Part model, mm, in its own coordinate system. Coordinates: 2 decimals unless noted, no trailing zeros. Order: outer loops, then holes, each group sorted by start corner. A loop starts at its lowest first (then second) coordinate and runs counter-clockwise, first axis right, second up.
1) Cut at C-C (z = 2). List the corners of the cut face in (x, y).
2) Cut at A-A (x = 0). List the corners of the cut face in (y, z), and give its area (3 significant figures).
3) Cut at D-D (y = -37.5). List the corners of the cut face in (x, z).
4) Pin check, flat tips, straight feed: pin 1 Ø3 at (x, z) = (-47.5, 5) entering from -Y (3 decimals); pin 2 Ø15 at (x, y) = (-76.2, 0) entering from +Z; pin 3 Ø3 at (x, z) = (31.5, 1) entering from -Y. Stop position of each tip, or through.
5) Cut at B-B (y = -4.5). List the corners of the cut face in (x, z).
6) Wall check: L1, parallel to Y at x = 0, z = 2.25; L2, parallel to X at y = 8.5, z = 5; L3, parallel to Y at x = -76.2, z = 4. Give the ranges that are in metal, low to high.
7) Mould opens along Y. For faces 1 (the cylindrical face through (-59.56, -34.48, 3.13)), 2 (the cylindrical face through (-59.14, 34.65, 3.13)), 3 (the flat face through (26, -41, 6.35)), 4 (the cylindrical face through (-64.086, 3.815, 3.131)) say: +Y half, -Y half, draft (parallel to the pull), parting line (faces both ways), or undercut.
```python
from build123d import *

# Parameters (mm, degrees)
F0_R     = 12.7
F0_R_2   = 44.45
F1_DEPTH = 6.35


# Not quite as in the source:
# - a length typed as a fraction of an inch, garbled in the dataset ("3 / 203.2 mm" for 3/8 in), is restored


with BuildPart() as f1:
    # F0 (on Top) → F1 (new body)
    with BuildSketch(Plane.XY):
        with BuildLine():
            ThreePointArc((-46.13671875, 43.6308741946), (-59.3475236203, 34.5646316236), (-75.1176136364, 31.7315448688))
            ThreePointArc((-75.1176136364, 31.7315448688), (-107.95, 0), (-75.1176136364, -31.7315448688))
            ThreePointArc((-75.1176136364, -31.7315448688), (-59.3475236203, -34.5646316236), (-46.13671875, -43.6308741946))
            ThreePointArc((-46.13671875, -43.6308741946), (-0.5192783502, -63.4978767361), (45.4169792735, -44.3795898321))
            ThreePointArc((45.4169792735, -44.3795898321), (60.1682182179, -35.0158685824), (77.5480268965, -33.2212721562))
            ThreePointArc((77.5480268965, -33.2212721562), (113.3582561105, -2.4068513639), (78.8882291033, 29.8997777276))
            ThreePointArc((78.8882291033, 29.8997777276), (61.6002556172, 32.4304493339), (47.2597573079, 42.4118537581))
            ThreePointArc((47.2597573079, 42.4118537581), (0.8287379603, 63.4945918437), (-46.13671875, 43.6308741946))
        make_face()
        with Locations((81.6154102788, -1.7328791769)):
            Circle(F0_R, mode=Mode.SUBTRACT)
        with Locations((-76.2, 0)):
            Circle(F0_R, mode=Mode.SUBTRACT)
        Circle(F0_R_2, mode=Mode.SUBTRACT)
    extrude(amount=F1_DEPTH)


solid = f1.part
```
Geometry check:
1. outline: (-75.12, -31.73) arc R38.1 cw to (-46.14, -43.63) arc R63.5 ccw to (45.42, -44.38) arc R38.1 cw to (77.55, -33.22) arc R31.75 ccw (long way) to (78.89, 29.9) arc R38.1 cw to (47.26, 42.41) arc R63.5 ccw to (-46.14, 43.63) arc R38.1 cw to (-75.12, 31.73) arc R31.75 ccw (long way) to start; hole circle Ø25.4 at (-76.2, 0); hole circle Ø88.9 at (0, 0); hole circle Ø25.4 at (81.62, -1.73)
2. outline: (-63.5, 0) - (-44.45, 0) - (-44.45, 6.35) - (-63.5, 6.35) - close; (44.45, 0) - (63.5, 0) - (63.5, 6.35) - (44.45, 6.35) - close
2. area: 242 mm2
3. outline: (-53.63, 0) - (-23.87, 0) - (-23.87, 6.35) - (-53.63, 6.35) - close; (23.87, 0) - (54.53, 0) - (54.53, 6.35) - (23.87, 6.35) - close
4. pin 1: stops at y = -43.775
4. pin 2: passes through
4. pin 3: stops at y = -55.97
5. outline: (-107.63, 0) - (-88.08, 0) - (-88.08, 6.35) - (-107.63, 6.35) - close; (-64.32, 0) - (-44.22, 0) - (-44.22, 6.35) - (-64.32, 6.35) - close; (44.22, 0) - (69.22, 0) - (69.22, 6.35) - (44.22, 6.35) - close; (94.01, 0) - (113.24, 0) - (113.24, 6.35) - (94.01, 6.35) - close
6. L1: y = -63.5 to -44.45, 44.45 to 63.5
6. L2: x = -106.79 to -85.64, -66.76 to -43.63, 43.63 to 74.09, 89.14 to 111.67
6. L3: y = -31.75 to -12.7, 12.7 to 31.75
7. face 1: -Y half
7. face 2: +Y half
7. face 3: draft
7. face 4: undercut
